Input: part model. Units: mm. Frame: model coordinates. A direction names the side the tool comes from. Round coordinates to 2 decimals unless told otherwise and drop trailing zeros. Order: outer loops, then holes, each group sorted by start corner. A loop starts at its lowest first (then second) coordinate and runs counter-clockwise, first axis right, second up.
Item 1: Cut plane A-A on x = 0. Output: boundary loops of the cut face in (y, z), then the cut area to 3 significant figures.
Item 2: Cut plane B-B on z = 58. Output: boundary loops of the cut face in (x, y), then the cut area to 3 significant figures.
Item 3: Line query: L1, parallel to Z at x = -50, y = -56; L2, parallel to X at y = 0, z = 59.5; L3, parallel to Y at x = 0, z = 54. Output: solid intervals per line, ascending.
Item 4: Cut plane D-D on x = -36. Output: boundary loops of the cut face in (y, z), then the cut area to 3 significant figures.
Item 5: Reachability of faces 4 (the flat face through (-52, -57, 75)), 5 (the cylindrical face through (34.765, -54.218, 37.04)), 6 (the flat face through (-50, -55, 37)) from +Z, -Z, +X, -X, +Y, -Y: full face, straight path, thin tool, end or side. Return the list, or none.
Item 6: Mould query, pull axis Y, two halves, no side actions, for faces 1 (the cylindrical face through (-11.164, -50.275, 105.929)), 2 (the cylindrical face through (0, -59, 37)), 3 (the cylindrical face through (-46.51, -57.46, 67.08)). Classes: released by +Y, released by -Y, zero draft, split by the parting line, or undercut.
Item 7: Cut plane C-C on y = -15. Output: boundary loops of the cut face in (x, z).
Item 8: First-contact query: pin 1 (6 mm diameter, centred on x = -22.5, z = 90.5, fed in from -Y); pin 2 (1.5 mm diameter, centred on x = 52.5, y = -56.5, fed in from +Z); pin 3 (6 mm diameter, centred on y = -10, z = 92.5, fed in from -X). Flat tips, straight axial feed; report the tip coordinate or a pass-through.
```python
from build123d import *

# Parameters (mm, degrees)
ESQUISSE1_R                     = 54
ESQUISSE1_R_2                   = 49
EXTRUSION1_DEPTH                = 108
ESQUISSE2_R                     = 51.5
ENL_V_MAT_EXTRU_1_DEPTH         = 4.2
ENL_V_START                     = -4.2
ESQUISSE3_R                     = 51.5
ENL_V_MAT_EXTRU_2_DEPTH         = 4.2
ESQUISSE4_W                     = 13.403361345
ESQUISSE4_H                     = 3
ENL_V_MAT_EXTRU_3_DEPTH         = 4.2
EXTRUSION2_DEPTH                = 75
ENL_V_MAT_EXTRU_4_REACH         = 170.286
ENL_V_MAT_EXTRU_4_END_RADIUS    = 54
EXTRUSION3_DEPTH                = 55
R_P_TITION_LIN_AIRE1_COUNT      = 2
R_P_TITION_LIN_AIRE1_PITCH      = 55
R_P_TITION_LIN_AIRE1_COUNT_DIR2 = 2
R_P_TITION_LIN_AIRE1_PITCH_DIR2 = 101


with BuildPart() as part:
    # Esquisse1 → Extrusion1 (new body)
    with BuildSketch(Plane.XY):
        Circle(ESQUISSE1_R)
        Circle(ESQUISSE1_R_2, mode=Mode.SUBTRACT)
    extrude(amount=EXTRUSION1_DEPTH)

    # Esquisse2 → Enlèv. mat.-Extru.1 (cut)
    with BuildSketch(Plane.XY.offset(108)):
        Circle(ESQUISSE2_R)
    extrude(amount=-ENL_V_MAT_EXTRU_1_DEPTH, mode=Mode.SUBTRACT)

    # Esquisse3 → Enlèv. mat.-Extru.2 (cut)
    with BuildSketch(Plane(origin=(0, 0, 0), x_dir=(-1, 0, 0), z_dir=(0, 0, -1)).offset(ENL_V_START)):
        with Locations(Location((0, 0, 0), (0, 0, 180))):
            Circle(ESQUISSE3_R)
    extrude(amount=ENL_V_MAT_EXTRU_2_DEPTH, mode=Mode.SUBTRACT)

    # Esquisse4 → Enlèv. mat.-Extru.3 (cut)
    with BuildSketch(Plane(origin=(0, 0, 0), x_dir=(-1, 0, 0), z_dir=(0, 0, -1))):
        with Locations((51.37955182, 0)):
            Rectangle(ESQUISSE4_W, ESQUISSE4_H)
    extrude(amount=-ENL_V_MAT_EXTRU_3_DEPTH, mode=Mode.SUBTRACT)

    # Esquisse5 → Extrusion2 (add)
    with BuildSketch(Plane(origin=(0, 0, 0), x_dir=(-1, 0, 0), z_dir=(0, 0, -1))):
        with BuildLine():
            Line((-60.5, -60), (-38.642135624, -60))
            ThreePointArc((-38.642135624, -60), (-32.901884138, -58.858192988), (-28.035533906, -55.606601718))
            Line((-28.035533906, -55.606601718), (-26.581131511, -54.152199323))
            ThreePointArc((-26.581131511, -54.152199323), (-25.525097055, -53.598747333), (-24.341773098, -53.744563283))
            ThreePointArc((-24.341773098, -53.744563283), (0, -59), (24.341773098, -53.744563283))
            ThreePointArc((24.341773098, -53.744563283), (25.525097055, -53.598747333), (26.581131511, -54.152199323))
            Line((26.581131511, -54.152199323), (28.035533906, -55.606601718))
            ThreePointArc((28.035533906, -55.606601718), (32.901884138, -58.858192988), (38.642135624, -60))
            Line((38.642135624, -60), (60.5, -60))
            Line((60.5, -60), (60.5, -55))
            Line((60.5, -55), (38.642135624, -55))
            ThreePointArc((38.642135624, -55), (34.8153013, -54.238795325), (31.571067812, -52.071067812))
            Line((31.571067812, -52.071067812), (30.116665417, -50.616665417))
            ThreePointArc((30.116665417, -50.616665417), (26.42054482, -48.67958345), (22.278910971, -49.189939276))
            ThreePointArc((22.278910971, -49.189939276), (0, -54), (-22.278910971, -49.189939276))
            ThreePointArc((-22.278910971, -49.189939276), (-26.42054482, -48.67958345), (-30.116665417, -50.616665417))
            Line((-30.116665417, -50.616665417), (-31.571067812, -52.071067812))
            ThreePointArc((-31.571067812, -52.071067812), (-34.8153013, -54.238795325), (-38.642135624, -55))
            Line((-38.642135624, -55), (-60.5, -55))
            Line((-60.5, -55), (-60.5, -60))
        make_face()
    extrude(amount=-EXTRUSION2_DEPTH)

    # Enlèv. mat.-Extru.4: up to this cylinder (the profile starts outside it)
    enl_v_mat_extru_4_end = Plane(origin=(0, 0, 37.5), z_dir=(0, 0, -1)) * Cylinder(ENL_V_MAT_EXTRU_4_END_RADIUS, 515.029516, mode=Mode.PRIVATE)
    # Esquisse6 → Enlèv. mat.-Extru.4 (cut, up to the surface)
    with BuildSketch(Plane.XZ.offset(60), mode=Mode.PRIVATE) as enl_v_mat_extru_4_sk1:
        Polygon((43.5, 0), (-43.5, 0), (-33, 10), (33, 10), align=None)
    enl_v_mat_extru_4_tool1 = extrude(enl_v_mat_extru_4_sk1.sketch, amount=-ENL_V_MAT_EXTRU_4_REACH, mode=Mode.PRIVATE) - enl_v_mat_extru_4_end
    add(enl_v_mat_extru_4_tool1.solids().sort_by_distance((0, -60, 4.771242))[0], mode=Mode.SUBTRACT)
    # Esquisse6 → Enlèv. mat.-Extru.4 (cut, up to the surface)
    with BuildSketch(Plane.XZ.offset(60), mode=Mode.PRIVATE) as enl_v_mat_extru_4_sk2:
        Polygon((-33, 65), (-43.5, 75), (43.5, 75), (33, 65), align=None)
    enl_v_mat_extru_4_tool2 = extrude(enl_v_mat_extru_4_sk2.sketch, amount=-ENL_V_MAT_EXTRU_4_REACH, mode=Mode.PRIVATE) - enl_v_mat_extru_4_end
    add(enl_v_mat_extru_4_tool2.solids().sort_by_distance((0, -60, 70.228758))[0], mode=Mode.SUBTRACT)

    # Esquisse7 → Extrusion3 (add)
    with BuildSketch(Plane(origin=(0, 0, 10), x_dir=(-1, 0, 0), z_dir=(0, 0, -1))):
        with BuildLine():
            Line((27.857974208, -46.259412804), (27.857974208, -49.104353136))
            ThreePointArc((27.857974208, -49.104353136), (25.059546429, -48.567236408), (22.278910971, -49.189939276))
            ThreePointArc((22.278910971, -49.189939276), (25.111228768, -47.806131299), (27.857974208, -46.259412804))
        make_face()
        with BuildLine():
            Line((-27.857974208, -46.259412804), (-27.857974208, -49.104353136))
            ThreePointArc((-27.857974208, -49.104353136), (-25.059546429, -48.567236408), (-22.278910971, -49.189939276))
            ThreePointArc((-22.278910971, -49.189939276), (-25.111228768, -47.806131299), (-27.857974208, -46.259412804))
        make_face()
    extrude(amount=-EXTRUSION3_DEPTH)

    # Esquisse10 → Dégagement M81 (revolve, cut)
    with BuildSketch(Plane(origin=(50.5, -55, 10), x_dir=(0, 0, 1), z_dir=(1, 0, 0))):
        Polygon((0, 0), (0, 26.703872786), (4.5, 24), (4.5, 0), align=None)
    d_gagement_m81 = revolve(axis=Axis((50.5, -48.65, 10), (0, -1, 0)), mode=Mode.SUBTRACT)

    # Répétition linéaire1: D_gagement M81 2 × 2
    with Locations(*[(-j * R_P_TITION_LIN_AIRE1_PITCH_DIR2, 0, i * R_P_TITION_LIN_AIRE1_PITCH) for i in range(R_P_TITION_LIN_AIRE1_COUNT) for j in range(R_P_TITION_LIN_AIRE1_COUNT_DIR2) if (i, j) != (0, 0)]):
        add(d_gagement_m81, mode=Mode.SUBTRACT)


solid = part.part
```
From the geometry:
1. outline: (-59, 10) - (-54, 10) - (-54, 0) - (-51.5, 0) - (-51.5, 4.2) - (-49, 4.2) - (-49, 103.8) - (-51.5, 103.8) - (-51.5, 108) - (-54, 108) - (-54, 65) - (-59, 65) - close; (49, 4.2) - (51.5, 4.2) - (51.5, 0) - (54, 0) - (54, 108) - (51.5, 108) - (51.5, 103.8) - (49, 103.8) - close
1. area: 1,310 mm2
2. outline: (-60.5, -60) - (-38.64, -60) arc R15 ccw to (-28.04, -55.61) - (-26.58, -54.15) arc R2 cw to (-24.34, -53.74) arc R59 ccw to (24.34, -53.74) arc R2 cw to (26.58, -54.15) - (28.04, -55.61) arc R15 ccw to (38.64, -60) - (60.5, -60) - (60.5, -55) - (38.64, -55) arc R10 cw to (31.57, -52.07) - (30.12, -50.62) arc R7 ccw to (27.86, -49.1) - (27.86, -46.26) arc R54 ccw (long way) to (-27.86, -46.26) - (-27.86, -49.1) arc R7 ccw to (-30.12, -50.62) - (-31.57, -52.07) arc R10 cw to (-38.64, -55) - (-60.5, -55) - close; hole circle Ø98 at (0, 0)
2. area: 2,260 mm2
3. L1: z = 0 to 5.53, 14.47 to 60.53, 69.47 to 75
3. L2: x = -54 to -49, 49 to 54
3. L3: y = -59 to -49, 49 to 54
4. outline: (-59.77, 7.14) - (-54.64, 7.14) - (-54.64, 67.86) - (-59.77, 67.86) - close; (-40.25, 0) - (-36.83, 0) - (-36.83, 4.2) - (-33.24, 4.2) - (-33.24, 103.8) - (-36.83, 103.8) - (-36.83, 108) - (-40.25, 108) - close; (33.24, 4.2) - (36.83, 4.2) - (36.83, 0) - (40.25, 0) - (40.25, 108) - (36.83, 108) - (36.83, 103.8) - (33.24, 103.8) - close
4. area: 1,760 mm2
5. face 4: +Z, +X, -X, -Y
5. face 5: +Z, -Z, +X
5. face 6: +Z, -Z, -X
6. face 1: undercut
6. face 2: released by -Y
6. face 3: zero draft
7. outline: (-51.87, 0) - (-49.27, 0) - (-49.27, 4.2) - (-46.65, 4.2) - (-46.65, 103.8) - (-49.27, 103.8) - (-49.27, 108) - (-51.87, 108) - close; (46.65, 4.2) - (49.27, 4.2) - (49.27, 0) - (51.87, 0) - (51.87, 108) - (49.27, 108) - (49.27, 103.8) - (46.65, 103.8) - close
8. pin 1: stops at y = -50.36
8. pin 2: stops at z = 75
8. pin 3: stops at x = -53.54
